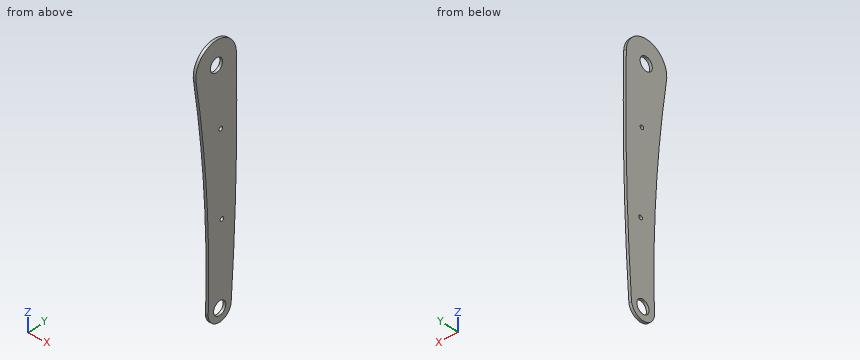
```python
from build123d import *

# Parameters (mm, degrees)
SKETCH_1_R      = 3.85
SKETCH_1_R_2    = 1.149031008
EXTRUDE_1_DEPTH = 1.5


with BuildPart() as part:
    # 草圖1 → 填料-伸長1 (new body)
    with BuildSketch(Plane(origin=(0, 0, 0), x_dir=(0, 0, -1), z_dir=(1, 0, 0))):
        with BuildLine():
            ThreePointArc((66.587683924, -5.116627236), (3.80507147, -6.050846657), (-58.633451622, -12.681082444))
            ThreePointArc((-58.633451622, -12.681082444), (-73.821962275, -1.715080477), (-61.804017134, 12.655481431))
            ThreePointArc((-61.804017134, 12.655481431), (3.033906142, 12.458288366), (67.798504291, 9.369274541))
            ThreePointArc((67.798504291, 9.369274541), (73.912446594, 1.807845069), (67.095645487, -5.12661445))
            ThreePointArc((67.095645487, -5.12661445), (66.8414518, -5.132449469), (66.587683924, -5.116627236))
        make_face()
        with Locations((66.61714054, 2.16157088)):
            Circle(SKETCH_1_R, mode=Mode.SUBTRACT)
        with Locations((-60.969663313, 0.079585479)):
            Circle(SKETCH_1_R, mode=Mode.SUBTRACT)
        with Locations((20.89210292, 3.571177524)):
            Circle(SKETCH_1_R_2, mode=Mode.SUBTRACT)
        with Locations((-26.521912025, 2.797466734)):
            Circle(SKETCH_1_R_2, mode=Mode.SUBTRACT)
    extrude(amount=EXTRUDE_1_DEPTH)


solid = part.part
```
Could you check a few things on this model? Use its own coordinates, in mm. Round coordinates to 2 decimals unless told otherwise and drop trailing zeros. Loops run counter-clockwise (first coordinate to the right, second up) from the corner with the lowest first, then second, coordinate; pieces in that order, holes last. Notation, with made-up numbers: M 19.25,59 L 78.25,59 A35 cw 78.25,97 Z; hole C 47,31.5 d11. An arc over 180 degrees is marked long. Put each result on its own line as item: value.
Q1. For pin 1 (4 mm diameter, centred on y = 7, z = -37.5, fed in from -X), with a flat end and sliding along its axis, tell me the tip position at first contact or that it passes through.
Check result:
pin 1: x = 0
Q2. Imagine slicing it at C-C (z = -4). Write out the boundary of the cut face in (x, y).
Check result:
outline: M 0,-6.04 L 1.5,-6.04 L 1.5,12.43 L 0,12.43 Z
Q3. Imagine slicing it at B-B (z = 52). Write out the boundary of the cut face in (x, y).
Check result:
outline: M 0,-11.7 L 1.5,-11.7 L 1.5,12.81 L 0,12.81 Z
Q4. I need wall thicknesses on probe 1 along Z at (x, y) = (0.5, 3.5); probe 2 along Y at (x, z) = (1, 59); probe 3 along Z at (x, y) = (1.1, 5.5). Which ranges of each line are inside material? Lowest first, please.
Check result:
probe 1: -73.8 to -70.23, -63.01 to -22.04, -19.75 to 25.61, 27.43 to 59.2, 62.74 to 73.4
probe 2: -12.75 to -3.23, 3.39 to 12.71
probe 3: -73.11 to -68.53, -64.7 to 72.62
Q5. Imagine slicing it at A-A (x = 0.75). Write out the boundary of the cut face in (y, z).
Check result:
outline: M -12.68,58.63 A690.9 cw -5.12,-66.59 A2.98 ccw -5.13,-67.1 A7.3 ccw 9.37,-67.8 A1453.29 ccw 12.66,61.8 A12.8 ccw long Z; hole C 0.08,60.97 d7.7; hole C 2.16,-66.62 d7.7; hole C 2.8,26.52 d2.3; hole C 3.57,-20.89 d2.3
